Job drawing, mm, ordinate dimensions from the low corner. One solid piece. Give positions to 0.01 mm unless a question says otherwise; leave off trailing zeros. Write each loop counter-clockwise with the first axis right and the second up, starting at its lowest first coordinate (ties: lowest second). Pieces come first, ordered by that corner, then holes. Notation, with made-up numbers: (1.25, 11.5) - (14.25, 11.5) arc R26 cw to (14.25, 45.5) - close; hole circle Ø8 at (39, 60). An arc over 180 degrees is marked (long way). Answer in a Markdown table with one row per item. Add a question column.
1. Band-saw the part on C-C on x = 69.5. Write the cut outline in (y, z), plus the area to 3 significant figures.
2. Band-saw the part on A-A on z = 7.85. Write the cut outline in (x, y).
3. Band-saw the part on B-B on x = 115.25. Write the cut outline in (y, z), plus the area to 3 significant figures.
4. Band-saw the part on D-D on z = 18. Write the cut outline in (x, y), plus the area to 3 significant figures.
5. Drop flat-ended pins along their axis: pin 1 Ø2 at (x, y) = (75.5, 0.5) entering from +Z; pin 2 Ø0.6 at (y, z) = (1.5, 59.5) entering from +X; pin 3 Ø1.6 at (x, y) = (72, 1) entering from -Z; pin 4 Ø2 at (x, z) = (2.25, 63.25) entering from -Y. Give the stop position or say it passes through.
6. Probe line 1 along Z through (x, y) = (115.25, 2.5); line 2 along X through (y, z) = (3.05, 7.85); line 3 along Y through (x, z) = (80, 49). List the from-to ranges inside material, lowest first.
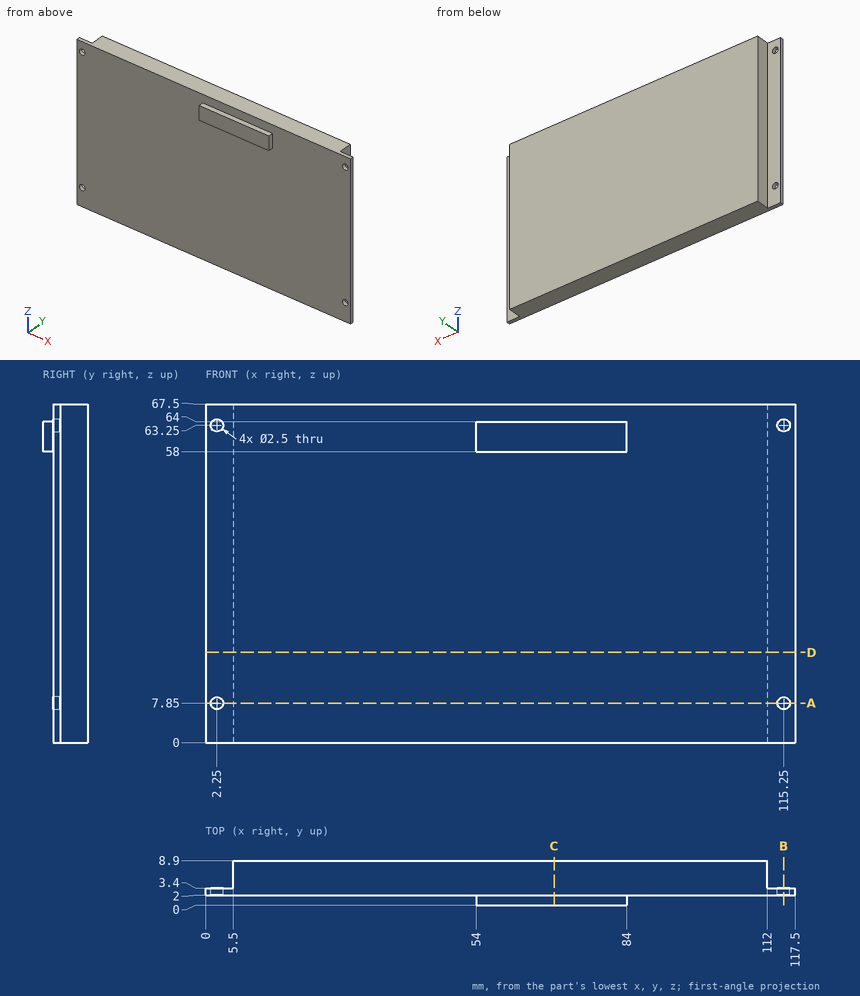
Values:
| question | item | result |
|---|---|---|
| 1 | outline | (0, 58) - (2, 58) - (2, 0) - (8.9, 0) - (8.9, 67.5) - (2, 67.5) - (2, 64) - (0, 64) - close |
| 1 | area | 478 mm² |
| 2 | outline | (0, 2) - (1, 2) - (1, 3.4) - (0, 3.4) - close; (3.5, 2) - (114, 2) - (114, 3.4) - (112, 3.4) - (112, 8.9) - (5.5, 8.9) - (5.5, 3.4) - (3.5, 3.4) - close; (116.5, 2) - (117.5, 2) - (117.5, 3.4) - (116.5, 3.4) - close |
| 3 | outline | (2, 0) - (3.4, 0) - (3.4, 6.6) - (2, 6.6) - close; (2, 9.1) - (3.4, 9.1) - (3.4, 62) - (2, 62) - close; (2, 64.5) - (3.4, 64.5) - (3.4, 67.5) - (2, 67.5) - close |
| 3 | area | 87.5 mm² |
| 4 | outline | (0, 2) - (117.5, 2) - (117.5, 3.4) - (112, 3.4) - (112, 8.9) - (5.5, 8.9) - (5.5, 3.4) - (0, 3.4) - close |
| 4 | area | 750 mm² |
| 5 | pin 1 | stops at z = 64 |
| 5 | pin 2 | stops at x = 84 |
| 5 | pin 3 | stops at z = 58 |
| 5 | pin 4 | passes through |
| 6 | line 1 | z = 0 to 6.6, 9.1 to 62, 64.5 to 67.5 |
| 6 | line 2 | x = 0 to 1, 3.5 to 114, 116.5 to 117.5 |
| 6 | line 3 | y = 2 to 8.9 |
